Can you work these out from the drawing? Everything is in mm from the part's minimum corner. Give positions to 0.01 mm unless a question says otherwise; leave off trailing zeros. Write each loop counter-clockwise with the first axis right and the second up, starting at its lowest first coordinate (ties: lowest second). Pieces come first, ordered by that corner, then holes. Notation, with made-up numbers: (-4, 35) - (20, 35) arc R20 cw to (20, 62) - close; hole circle Ø5 at (45.5, 20). An arc over 180 degrees is marked (long way). Use a Markdown table: item, result.
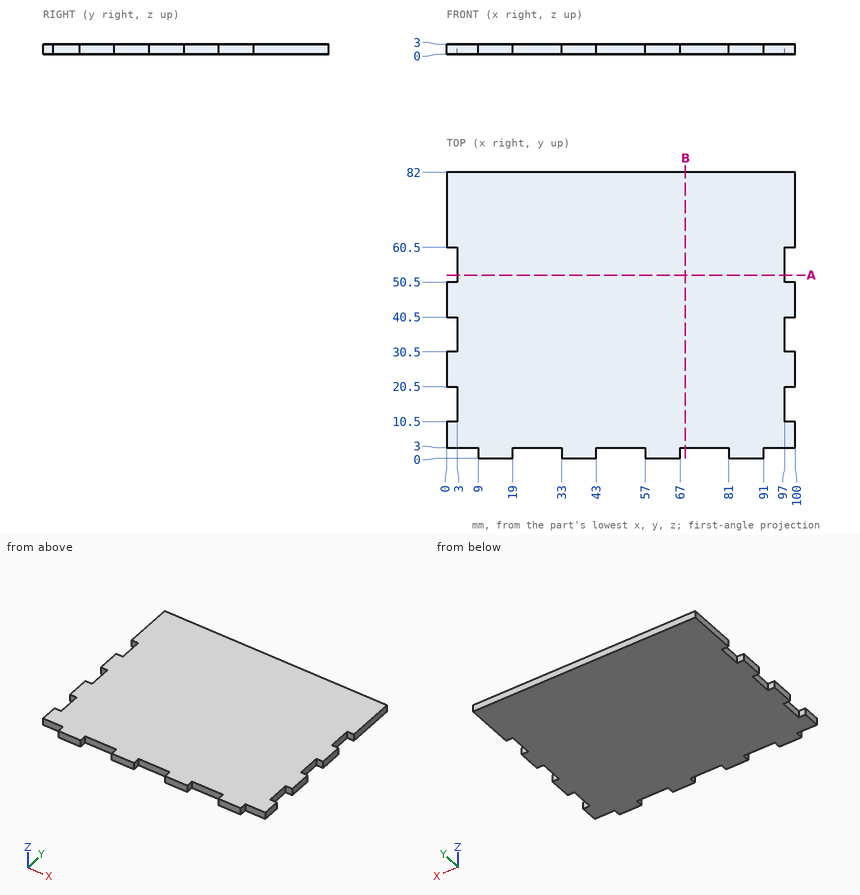
Item 1: If we section it at A-A, the plane y = 52.5: Write out the boundary of the cut face in (x, z).
Values:
| item | result |
|---|---|
| outline | (3, 0) - (97, 0) - (97, 3) - (3, 3) - close |
Item 2: I need wall thicknesses on line 1 along X through (y, z) = (16.5, 0.2); line 2 along Y through (x, z) = (53, 2.8). Which ranges of each line are inside material? Lowest first, please. Write a range as [from, to].
Values:
| item | result |
|---|---|
| line 1 | x = [3, 97] |
| line 2 | y = [3, 82] |
Item 3: Will these pins go through, and if not, where does the flat tip stop? pin 1 Ø0.9 at (y, z) = (2, 1.5) entering from +X; pin 2 Ø1.5 at (y, z) = (33.5, 1) entering from -X; pin 3 Ø0.9 at (y, z) = (14, 2) entering from +X.
Values:
| item | result |
|---|---|
| pin 1 | stops at x = 91 |
| pin 2 | stops at x = 3 |
| pin 3 | stops at x = 97 |
Item 4: If we section it at B-B, the plane x = 68.5: Write out the boundary of the cut face in (y, z).
Values:
| item | result |
|---|---|
| outline | (3, 0) - (82, 0) - (82, 3) - (3, 3) - close |
